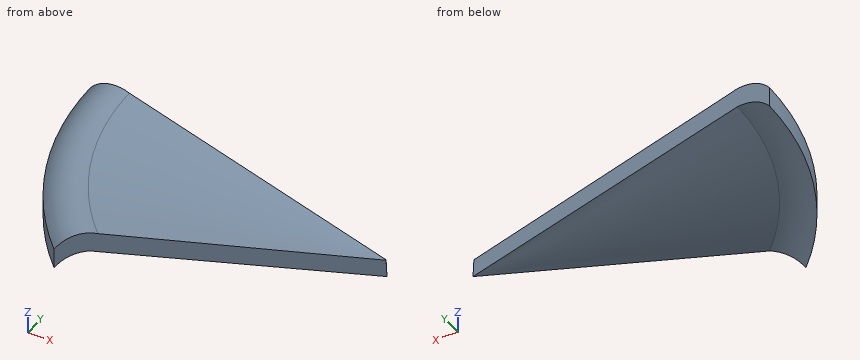
from build123d import *

# Parameters (mm, degrees)
F1_ANGLE = 45


# Not quite as in the source:
# - a feature names something its author has since deleted; it is built from what else it names


with BuildPart() as f1:
    # F0 (on Front) → F1 (revolve)
    with BuildSketch(Plane.XZ):
        with BuildLine():
            Line((0, 0), (-0.3200573587, 6.5955988818))
            Line((-0.3200573587, 6.5955988818), (-93.7548232766, 35.8510324721))
            ThreePointArc((-93.7548232766, 35.8510324721), (-101.4397958576, 36.5208008084), (-107.92452842, 32.3428064585))
            Line((-107.92452842, 32.3428064585), (-107.92452842, 24.9973144382))
            ThreePointArc((-107.92452842, 24.9973144382), (-102.6379346155, 28.7570956855), (-96.1832379704, 29.4058793942))
            Line((-96.1832379704, 29.4058793942), (0, 0))
        make_face()
    revolve(axis=Axis((0, 0, 59.7953810357), (0, 0, 1)), revolution_arc=F1_ANGLE)


solid = f1.part
CAD build for the part. Positions are in the model's coordinates, mm. Coordinates: 2 decimals unless noted, no trailing zeros. Loops run counter-clockwise (first coordinate to the right, second up) from the corner with the lowest first, then second, coordinate; pieces in that order, holes last. Notation, with made-up numbers: (45.25, 29) - (53.25, 29) arc R5 cw to (53.25, 35) - close; hole circle Ø2 at (-27, -7.5). An arc over 180 degrees is marked (long way). Write item = value, one per line. Start each with the question number.
Q1. Cut at A-A, the plane z = 4. List the corners of the cut face in (x, y).
Q2. Cut at B-B, the plane z = 21. List the corners of the cut face in (x, y), then the cut area to 3 significant figures.
Q3. Flat gauge pins, fed straight in: pin 1 Ø12 at (x, y) = (-55.5, -44) entering from -Z; pin 2 Ø8 at (x, y) = (-80.5, -64.5) entering from +Z; pin 3 Ø1.5 at (x, z) = (-47.5, 18.5) entering from +Y; pin 4 Ø5 at (y, z) = (-28, 17) entering from +X. Where does each tip first touch, or does it go through?
Q4. Drill centre lines: L1, parallel to Z at x = -72.5, y = -66; L2, parallel to Z at x = -30, y = -24; L3, parallel to X at y = -68, z = 35. Where is each one in solid material? Low to high.
Computed:
q1.outline = (-13.08, 0) arc R13.08 ccw to (-9.25, -9.25) - (-0.14, -0.14) arc R0.19 cw to (-0.19, 0) - close
q2.outline = (-68.69, 0) arc R68.69 ccw to (-48.57, -48.57) - (-32.76, -32.76) arc R46.32 cw to (-46.32, 0) - close
q2.area = 1,010 mm²
q3.pin_1 = 19.82
q3.pin_2 = 36.86
q3.pin_3 = 0
q3.pin_4 = -25.5
q4.L1 = 29.56 to 36.86
q4.L2 = 11.75 to 18.52
q4.L3 = -79.99 to -68
